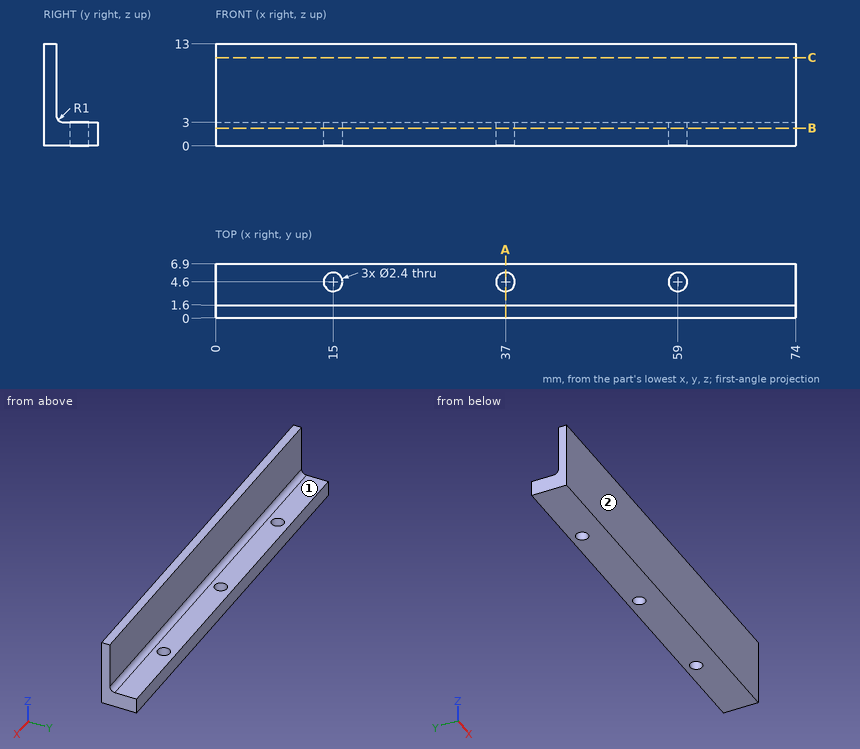
Geometry: see drawing. Coordinates: mm, zero at the bounding-box minimum. A direction names the side the tool comes from. Round coordinates to 2 decimals unless told otherwise and drop trailing zeros. Loops run counter-clockwise (first coordinate to the right, second up) from the corner with the lowest first, then second, coordinate; pieces in that order, holes last. Notation, with made-up numbers: (-35.5, 85) - (-1.5, 85) arc R32 cw to (-1.5, 111) - close; hole circle Ø6 at (67.25, 78). An arc over 180 degrees is marked (long way). One line per item, written item: value. Start each with the question number.
(1) Access query for the marked faces 1 and 2. Directions: +Z, -Z, +X, -X, +Y, -Y. A direction counts if a zero-diameter tool reaches every point of the face in a straight line with its end or side. Return the directions, or none.
(2) Section A-A, the plane x = 37. Return loops of the section in (y, z), plus the area to 3 significant figures.
(3) Section C-C, the plane z = 11.25. Return loops of the section in (x, y), plus the area to 3 significant figures.
(4) Section B-B, the plane z = 2.25. Return loops of the section in (x, y), plus the area to 3 significant figures.
(5) Ray query, line 1 (Y direction, x = 15, z = 1.85); line 2 (Z direction, x = 14.5, y = 2.5); line 3 (Y direction, x = 7, z = 10.5). Return the intervals inside material, ascending. Write a range as [from, to].
(6) Contact query for flat-ended pins moving along their axis: P1, Ø1, axis at x = 44.5, z = 7, coming from the -Y side; P2, Ø2.5, axis at x = 43, z = 9, coming from the +Y side; P3, Ø1.9, axis at x = 59, y = 4.6, coming from the +Z side; P4, Ø3, axis at x = 15, y = 4.6, coming from the +Z side. Output: stop coordinate, or through.
Results below:
1. face 1: +Z, +X, -X, +Y
1. face 2: +Z, -Z, +X, -X, -Y
2. outline: (0, 0) - (3.4, 0) - (3.4, 3) - (2.6, 3) arc R1 cw to (1.6, 4) - (1.6, 13) - (0, 13) - close; (5.8, 0) - (6.9, 0) - (6.9, 3) - (5.8, 3) - close
2. area: 29.7 mm^2
3. outline: (0, 0) - (74, 0) - (74, 1.6) - (0, 1.6) - close
3. area: 118 mm^2
4. outline: (0, 0) - (74, 0) - (74, 6.9) - (0, 6.9) - close; hole circle Ø2.4 at (15, 4.6); hole circle Ø2.4 at (37, 4.6); hole circle Ø2.4 at (59, 4.6)
4. area: 497 mm^2
5. line 1: [0, 3.4], [5.8, 6.9]
5. line 2: [0, 3.01]
5. line 3: [0, 1.6]
6. P1: y = 0
6. P2: y = 1.6
6. P3: through
6. P4: z = 3
